Check sheet for the modelled part. Datum: model origin and axes. Units: mm. A direction names the side the tool comes from. Coordinates: 2 decimals unless noted, no trailing zeros. Write each loop counter-clockwise with the first axis right and the second up, starting at its lowest first coordinate (ties: lowest second). Pieces come first, ordered by that corner, then holes. Notation, with made-up numbers: (27.25, 25.25) -> (86.25, 25.25) arc R22 ccw to (86.25, 52.25) -> close; hole circle Ø4 at (-2, 60). An arc over 180 degrees is marked (long way). One line per item, written item: value. Start each with the question number.
1) Sectioned sample at A-A on x = 5. Enter the section's corners in (y, z), plus the area to 3 significant figures.
2) Sectioned sample at B-B on y = 31. Enter the section's corners in (x, z), plus the area to 3 significant figures.
3) Gauge pin test, flat ends, axial feed: P1, Ø5, axis at x = 60, y = 13.5, coming from the +Z side; P2, Ø1.6, axis at y = 33.5, z = 0.5, coming from the +X side; P3, Ø16, axis at x = 58.5, y = 32.5, coming from the -Z side; P4, Ø3, axis at x = 60, y = 13.5, coming from the -Z side. Record the tip position at first contact, or that the pin passes through.
4) Draft check along X on faces 1 (the flat face through (42, 31, 6)), 2 (the cylindrical face through (0.57, 0.6, 3.04)), 3 (the cylindrical face through (5.8, 32.5, 3)), 4 (the flat face through (39.5, 31, 3)). Enter one of: +X half, -X half, draft (parallel to the pull), parting line (faces both ways), or undercut.
5) Scan lines: line 1 along Y through (x, z) = (60, 3.7); line 2 along Y through (x, z) = (60, 5.55); line 3 along X through (y, z) = (37, 0.3). Record each from-to range of solid material in increasing order. Write a range as [from, to].
6) Sectioned sample at D-D on x = 60. Enter the section's corners in (y, z).
7) Sectioned sample at C-C on z = 3.4. Enter the section's corners in (x, y).
8) Set-up check for faces 5 (the flat face through (35, 0, 3)), 6 (the cylindrical face through (57, 13.6, 5.3)), 7 (the flat face through (10.5, 31, 3)), 8 (the flat face through (60, 31, 2)), 9 (the flat face through (70, 31, 4)): record each of +Z, -Z, +X, -X, +Y, -Y from which the full face is reachable in a straight line by a thin tool's end or side.
Autodesk Inventor part; units mm, degrees
ref_plane "YZ Plane" through (0, 0, 0) normal (1, 0, 0) x (0, 1, 0)
ref_plane "XZ Plane" through (0, 0, 0) normal (0, 1, 0) x (-1, 0, 0)
ref_plane "XY Plane" through (0, 0, 0) normal (0, 0, 1) x (1, 0, 0)
sketch "Sketch1" plane through (0, 0, 0) normal (0, 0, 1) x (1, 0, 0)
  line L0 (0, 0) -> (50, 0)
  line L1 (50, 0) -> (50, 62)
  line L2 (50, 62) -> (0, 62)
  line L3 (0, 62) -> (0, 0)
  circle A0 centre (5, 31) radius 1.7
  circle A1 centre (45, 31) radius 1.7
  line L4 (10.5, 55.5) -> (39.5, 55.5)
  line L5 (39.5, 55.5) -> (39.5, 6.5)
  line L6 (39.5, 6.5) -> (10.5, 6.5)
  line L7 (10.5, 6.5) -> (10.5, 55.5)
  line L8 (25, 55.5) -> (25, 6.5) construction
  point P0 (10.5, 31)
  point P1 (39.5, 31)
  point P2 (50, 31)
  dimension "d0" = 3.4
  dimension "d1" = 3.4
  dimension "d2" = 40
  dimension "d3" = 29
  dimension "d4" = 49
  dimension "d5" = 5
  dimension "d6" = 5
  dimension "d7" = 62
extrude "Extrusion1" add sketch "Sketch1" along normal blind 6
sketch "Sketch3" plane through (0, 0, 6) normal (0, 0, 1) x (1, 0, 0)
  line L0 (50, 62) -> (0, 62)
  line L1 (50, 62) -> (70, 62)
  line L2 (70, 62) -> (70, 0)
  line L3 (70, 0) -> (50, 0)
  line L4 (50, 0) -> (50, 62)
  circle A0 centre (60, 48.5) radius 1.7
  circle A1 centre (60, 13.5) radius 1.7
  line L5 (60, 48.5) -> (60, 13.5) construction
  point P0 (0, 0)
  point P1 (60, 0)
  point P2 (60, 31)
  point P3 (70, 31)
  dimension "d14" = 20
  dimension "d15" = 3.4
  dimension "d16" = 3.4
  dimension "d17" = 35
extrude "Extrusion3" add sketch "Sketch3" against normal blind 4
sketch "Sketch4" plane through (0, 0, 6) normal (0, 0, 1) x (1, 0, 0)
  circle A0 centre (60, 48.5) radius 1.7
  circle A1 centre (60, 13.5) radius 1.7
  circle A2 centre (60, 48.5) radius 1.7
  circle A3 centre (60, 48.5) radius 3
  circle A4 centre (60, 13.5) radius 1.7
  circle A5 centre (60, 13.5) radius 3
  point P0 (0, 0)
  dimension "d20" = 6
  dimension "d21" = 6
extrude "Extrusion4" cut sketch "Sketch4" against normal blind 1.5
fillet "Fillet1" radius 2 4 edges at (0, 62, 3) (0, 0, 3) (70, 0, 4) (70, 62, 4)
properties part number "power_switch_bracket"
Answers:
1. outline: (0, 0) -> (29.3, 0) -> (29.3, 6) -> (0, 6) -> close; (32.7, 0) -> (62, 0) -> (62, 6) -> (32.7, 6) -> close
1. area: 352 mm2
2. outline: (0, 0) -> (3.3, 0) -> (3.3, 6) -> (0, 6) -> close; (6.7, 0) -> (10.5, 0) -> (10.5, 6) -> (6.7, 6) -> close; (39.5, 0) -> (43.3, 0) -> (43.3, 6) -> (39.5, 6) -> close; (46.7, 0) -> (50, 0) -> (50, 2) -> (70, 2) -> (70, 6) -> (46.7, 6) -> close
2. area: 165 mm2
3. P1: stops at z = 4.5
3. P2: stops at x = 50
3. P3: stops at z = 2
3. P4: passes through
4. face 1: draft
4. face 2: -X half
4. face 3: undercut
4. face 4: undercut
5. line 1: y = [0, 11.8], [15.2, 46.8], [50.2, 62]
5. line 2: y = [0, 10.5], [16.5, 45.5], [51.5, 62]
5. line 3: x = [0, 10.5], [39.5, 50]
6. outline: (0, 2) -> (11.8, 2) -> (11.8, 4.5) -> (10.5, 4.5) -> (10.5, 6) -> (0, 6) -> close; (15.2, 2) -> (46.8, 2) -> (46.8, 4.5) -> (45.5, 4.5) -> (45.5, 6) -> (16.5, 6) -> (16.5, 4.5) -> (15.2, 4.5) -> close; (50.2, 2) -> (62, 2) -> (62, 6) -> (51.5, 6) -> (51.5, 4.5) -> (50.2, 4.5) -> close
7. outline: (0, 2) arc R2 ccw to (2, 0) -> (68, 0) arc R2 ccw to (70, 2) -> (70, 60) arc R2 ccw to (68, 62) -> (2, 62) arc R2 ccw to (0, 60) -> close; hole circle Ø3.4 at (5, 31); hole (10.5, 6.5) -> (39.5, 6.5) -> (39.5, 55.5) -> (10.5, 55.5) -> close; hole circle Ø3.4 at (45, 31); hole circle Ø3.4 at (60, 13.5); hole circle Ø3.4 at (60, 48.5)
8. face 5: +Z, -Z, +X, -X, -Y
8. face 6: +Z
8. face 7: +Z, -Z
8. face 8: -Z, +X, +Y, -Y
8. face 9: +Z, -Z, +X, +Y, -Y
